Answer from the drawing. Dimensions are ordinates in mm from the lowest x, y and z of the part. Round coordinates to 2 decimals unless told otherwise and drop trailing zeros. Loops run counter-clockwise (first coordinate to the right, second up) from the corner with the lowest first, then second, coordinate; pieces in that order, holes last.
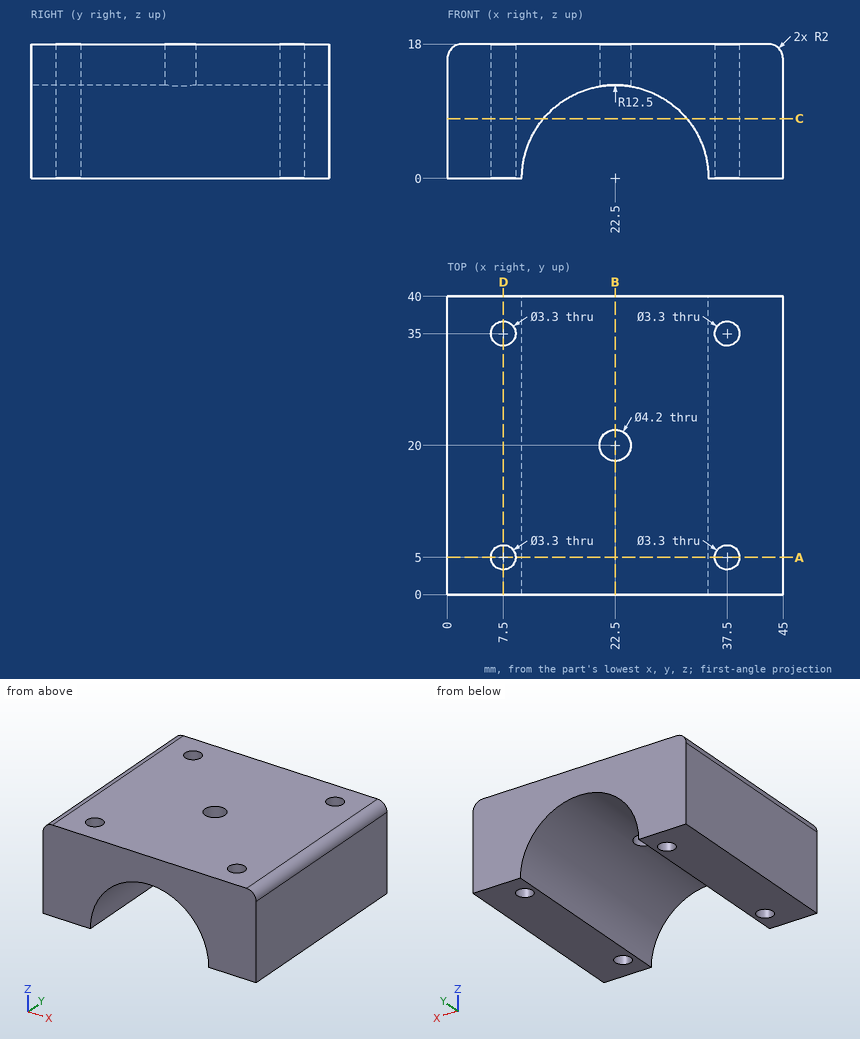
1. Consider probe 1 along Y at (x, z) = (7.5, 12.25); probe 2 along Y at (x, z) = (22.5, 14.6); probe 3 along X at (y, z) = (36.5, 9.25). Determine where each line is inside the solid, lowest interval first.
Answer key:
probe 1: y = 0 to 3.35, 6.65 to 33.35, 36.65 to 40
probe 2: y = 0 to 17.9, 22.1 to 40
probe 3: x = 0 to 6.81, 8.19 to 14.09, 30.91 to 36.81, 38.19 to 45
2. Find section A-A (y = 5). Write down the section's boundary in (x, z).
Answer key:
outline: (0, 0) - (5.85, 0) - (5.85, 18) - (2, 18) arc R2 ccw to (0, 16) - close; (9.15, 0) - (10, 0) arc R12.5 cw to (35, 0) - (35.85, 0) - (35.85, 18) - (9.15, 18) - close; (39.15, 0) - (45, 0) - (45, 16) arc R2 ccw to (43, 18) - (39.15, 18) - close
3. Given pin 1 (4.5 mm diameter, centred on x = 7.5, y = 35, fed in from +Z); pin 2 (5.5 mm diameter, centred on x = 22.5, y = 20, fed in from -Z), each flat-ended and moving along its own axis, determine where each tip first touches the part or whether it passes through.
Answer key:
pin 1: stops at z = 18
pin 2: stops at z = 12.19
4. Find section B-B (x = 22.5). Write down the section's boundary in (y, z), then the cut area to 3 significant figures.
Answer key:
outline: (0, 12.5) - (17.9, 12.5) - (17.9, 18) - (0, 18) - close; (22.1, 12.5) - (40, 12.5) - (40, 18) - (22.1, 18) - close
area: 197 mm2
5. Find section C-C (z = 8). Write down the section's boundary in (x, y).
Answer key:
outline: (0, 0) - (12.9, 0) - (12.9, 40) - (0, 40) - close; (32.1, 0) - (45, 0) - (45, 40) - (32.1, 40) - close; hole circle Ø3.3 at (7.5, 5); hole circle Ø3.3 at (7.5, 35); hole circle Ø3.3 at (37.5, 5); hole circle Ø3.3 at (37.5, 35)
6. Find section D-D (x = 7.5). Write down the section's boundary in (y, z).
Answer key:
outline: (0, 0) - (3.35, 0) - (3.35, 18) - (0, 18) - close; (6.65, 0) - (33.35, 0) - (33.35, 18) - (6.65, 18) - close; (36.65, 0) - (40, 0) - (40, 18) - (36.65, 18) - close
